from build123d import *

# Parameters (mm, degrees)
BOSS_EXTRUDE1_DEPTH     = 6.35
SKETCH2_R               = 1.5
CUT_EXTRUDE1_DEPTH      = 39.1
CUT_EXTRUDE1_DEPTH_BACK = 39.1


with BuildPart() as part:
    # Sketch1 → Boss-Extrude1 (new body)
    with BuildSketch(Plane(origin=(0, 0, 0), x_dir=(1, 0, 0), z_dir=(0, 1, 0))):
        Polygon((0, 0), (0, 12.7), (25.4, 60.325), (38.1, 60.325), (38.1, 107.95), (47.625, 107.95), (76.2, 12.7), (76.2, 0), align=None)
    extrude(amount=BOSS_EXTRUDE1_DEPTH)

    # Sketch2 → Cut-Extrude1 (cut, two sides)
    with BuildSketch(Plane.ZY.offset(-38.1)) as cut_extrude1_sk:
        with Locations((-101.6, 3.175)):
            Circle(SKETCH2_R)
        with Locations((-71.4375, 3.175)):
            Circle(SKETCH2_R)
    extrude(amount=CUT_EXTRUDE1_DEPTH, mode=Mode.SUBTRACT)
    extrude(cut_extrude1_sk.sketch, amount=-CUT_EXTRUDE1_DEPTH_BACK, mode=Mode.SUBTRACT)


solid = part.part
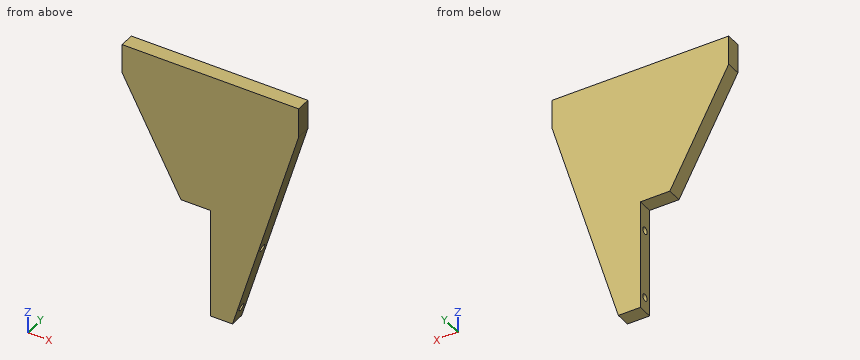
The listing builds one solid part. Answer for the finished solid, in the listing's coordinates (mm). Coordinates: 2 decimals unless noted, no trailing zeros. Write each loop counter-clockwise with the first axis right and the second up, starting at its lowest first coordinate (ties: lowest second). Pieces come first, ordered by that corner, then holes. Notation, with made-up numbers: (57, 52.5) - (80, 52.5) arc R27 ccw to (80, 69.5) - close; hole circle Ø3 at (37, -1.5). An arc over 180 degrees is marked (long way). Answer as CSV lines item,"result".
1. Straight lines are drawn through the part: line 1 (Y direction, x = 41.75, z = -101.6) (3 decimals); line 2 (Z direction, x = 46, y = 4.5); line 3 (Y direction, x = 46, z = -101). For each, find the intervals that lie inside material, in ascending order. Write a range as [from, to].
Computed values:
line 1,"y = [0, 1.675], [4.675, 6.35]"
line 2,"z = [-107.95, -102.3], [-100.9, -72.14], [-70.73, 0]"
line 3,"y = [0, 1.8], [4.55, 6.35]"
2. Find section D-D (z = -81). Give the vertices of the cut face in (x, y), plus the area to 3 significant figures.
Computed values:
outline,"(38.1, 0) - (55.71, 0) - (55.71, 6.35) - (38.1, 6.35) - close"
area,"112 mm²"
3. Find section A-A (z = -101.6). Give the vertices of the cut face in (x, y) (3 decimals), plus the area to 3 significant figures.
Computed values:
outline,"(38.1, 0) - (49.53, 0) - (49.53, 1.675) - (38.1, 1.675) - close; (38.1, 4.675) - (49.53, 4.675) - (49.53, 6.35) - (38.1, 6.35) - close"
area,"38.3 mm²"
4. Given P1, Ø1.9, axis at x = 34.5, y = 2, coming from the -Z side (3 decimals); P2, Ø1.9, axis at y = 3, z = -96, coming from the -X side; P3, Ø10, axis at x = 54, z = -77.5, coming from the -Y side, each flat-ended and moving along its own axis, determine where each tip first touches the part or whether it passes through.
Computed values:
P1,"stops at z = -60.325"
P2,"stops at x = 38.1"
P3,"stops at y = 0"
5. Find section C-C (x = 36.5). Give the vertices of the cut face in (y, z) (3 decimals), plus the area to 3 significant figures.
Computed values:
outline,"(0, -60.325) - (6.35, -60.325) - (6.35, 0) - (0, 0) - close"
area,"383 mm²"
